from build123d import *

# Parameters (mm, degrees)
CROQUIS1_W              = 42.3
CROQUIS1_H              = 42.3
SALIENTE_EXTRUIR1_DEPTH = 7.6
SKETCH1_R               = 29.910616844
SKETCH1_R_2             = 27
CUT_EXTRUDE1_DEPTH      = 8.6
CROQUIS3_R              = 11
CROQUIS3_R_2            = 8.5
SALIENTE_EXTRUIR2_DEPTH = 2
CROQUIS4_R              = 4.5
CORTAR_EXTRUIR2_DEPTH   = 7
CROQUIS5_R              = 2.5
CORTAR_EXTRUIR3_DEPTH   = 7
CROQUIS6_R              = 1.5
CORTAR_EXTRUIR4_DEPTH   = 4.5
SKETCH2_R               = 5.5
CUT_EXTRUDE2_DEPTH      = 7.1
SKETCH3_R               = 16.5
SKETCH3_R_2             = 11.5
CUT_EXTRUDE3_DEPTH      = 0.1
FILLET1_R               = 1
FILLET2_R               = 0.5
CHAMFER1_SIZE           = 0.5


with BuildPart() as part:
    # Croquis1 → Saliente-Extruir1 (new body)
    with BuildSketch(Plane.XY):
        Rectangle(CROQUIS1_W, CROQUIS1_H)
    extrude(amount=SALIENTE_EXTRUIR1_DEPTH)

    # Sketch1 → Cut-Extrude1 (cut, through all)
    with BuildSketch(Plane(origin=(0, 0, 0), x_dir=(-1, 0, 0), z_dir=(0, 0, -1))):
        Circle(SKETCH1_R)
        Circle(SKETCH1_R_2, mode=Mode.SUBTRACT)
    extrude(amount=-CUT_EXTRUDE1_DEPTH, mode=Mode.SUBTRACT)

    # Croquis3 → Saliente-Extruir2 (add)
    with BuildSketch(Plane(origin=(0, 0, 0), x_dir=(-1, 0, 0), z_dir=(0, 0, -1))):
        Circle(CROQUIS3_R)
        Circle(CROQUIS3_R_2, mode=Mode.SUBTRACT)
    extrude(amount=SALIENTE_EXTRUIR2_DEPTH)

    # Croquis4 → Cortar-Extruir2 (cut)
    with BuildSketch(Plane(origin=(0, 0, -2), x_dir=(-1, 0, 0), z_dir=(0, 0, -1))):
        Circle(CROQUIS4_R)
    extrude(amount=-CORTAR_EXTRUIR2_DEPTH, mode=Mode.SUBTRACT)

    # Croquis5 → Cortar-Extruir3 (cut)
    with BuildSketch(Plane(origin=(0, 0, 5), x_dir=(-1, 0, 0), z_dir=(0, 0, -1))):
        Circle(CROQUIS5_R)
    extrude(amount=-CORTAR_EXTRUIR3_DEPTH, mode=Mode.SUBTRACT)

    # Croquis6 → Cortar-Extruir4 (cut)
    with BuildSketch(Plane(origin=(0, 0, 0), x_dir=(-1, 0, 0), z_dir=(0, 0, -1))):
        with Locations((-15.5, 15.5)):
            Circle(CROQUIS6_R)
        with Locations((15.5, 15.5)):
            Circle(CROQUIS6_R)
        with Locations((15.5, -15.5)):
            Circle(CROQUIS6_R)
        with Locations((-15.5, -15.5)):
            Circle(CROQUIS6_R)
    extrude(amount=-CORTAR_EXTRUIR4_DEPTH, mode=Mode.SUBTRACT)

    # Sketch2 → Cut-Extrude2 (cut)
    with BuildSketch(Plane.XY.offset(7.6)):
        Circle(SKETCH2_R)
    extrude(amount=-CUT_EXTRUDE2_DEPTH, mode=Mode.SUBTRACT)

    # Sketch3 → Cut-Extrude3 (cut)
    with BuildSketch(Plane(origin=(0, 0, 0), x_dir=(-1, 0, 0), z_dir=(0, 0, -1))):
        Circle(SKETCH3_R)
        Circle(SKETCH3_R_2, mode=Mode.SUBTRACT)
    extrude(amount=-CUT_EXTRUDE3_DEPTH, mode=Mode.SUBTRACT)

    # Fillet1
    fillet1_edges = [part.edges().sort_by_distance(p)[0] for p in [
        (21.15, 16.783250579, 3.8),
        (21.15, -16.783250579, 3.8),
        (-16.783250579, 21.15, 3.8),
        (16.783250579, 21.15, 3.8),
        (-21.15, -16.783250579, 3.8),
        (-21.15, 16.783250579, 3.8),
        (16.783250579, -21.15, 3.8),
        (-16.783250579, -21.15, 3.8),
    ]]
    fillet(fillet1_edges, radius=FILLET1_R)

    # Fillet2
    fillet2_edges = [part.edges().sort_by_distance(p)[0] for p in [
        (19.091883092, 19.091883092, 0),
        (0, 21.15, 0),
        (-21.15, 0, 0),
        (-19.091883092, 19.091883092, 0),
        (21.15, 0, 0),
        (19.091883092, -19.091883092, 0),
        (0, -21.15, 0),
        (-19.091883092, -19.091883092, 0),
        (-16.766402254, 21.092072184, 0),
        (-21.092072184, 16.766402254, 0),
        (-21.092072184, -16.766402254, 0),
        (-16.766402254, -21.092072184, 0),
        (16.766402254, -21.092072184, 0),
        (21.092072184, -16.766402254, 0),
        (21.092072184, 16.766402254, 0),
        (16.766402254, 21.092072184, 0),
    ]]
    fillet(fillet2_edges, radius=FILLET2_R)

    # Chamfer1
    chamfer1_edges = [part.edges().sort_by_distance(p)[0] for p in [
        (11, 0, -2),
    ]]
    chamfer(chamfer1_edges, length=CHAMFER1_SIZE)


solid = part.part
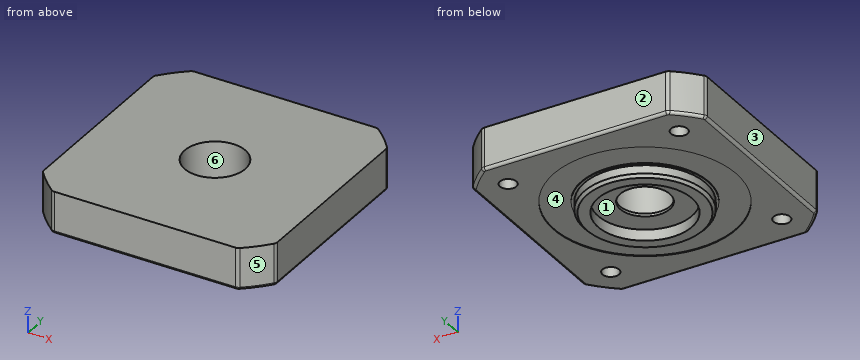
Could you check a few things on this model? Use its own coordinates, in mm. Face numbers are marked on the shaded views. A direction names the side the tool comes from. Give positions to 0.01 mm unless a question says otherwise; leave off trailing zeros. Order: outer loops, then holes, each group sorted by start corner. A loop starts at its lowest first (then second) coordinate and runs counter-clockwise, first axis right, second up. Notation, with made-up numbers: (11.25, -14.5) - (17.25, -14.5) arc R25 cw to (17.25, 17.5) - close; hole circle Ø5 at (58, 77.5). An arc over 180 degrees is marked (long way). One line per item, written item: value. Start each with the question number.
1. Imagine slicing it at C-C on y = -15. List the corners of the cut face in (x, z) for me, plus the area to 3 significant figures.
2. For P1, Ø8, axis at x = 0, y = 0, coming from the +Z side; P2, Ø2.5, axis at x = -16, y = -16, coming from the -Z side; P3, Ø2.5, axis at x = -15.5, y = -15.5, coming from the -Z side, each with a flat end and sliding along its axis, tell me the tip position at first contact or that it passes through.
3. For the marked faces 4, 5 and 6, which set-ups out of +Z, -Z, +X, -X, +Y, -Y let a thin tool reach every point of the face, with its end or its side?
4. Thinking about a two-plate mould opening in Y: for the marked faces 1, 2 and 3, which applies, +Y half, -Y half, draft (parallel to the pull), parting line (faces both ways), or undercut?
5. Imagine slicing it at D-D on z = -1. List the corners of the cut face in (x, y) for me.
6. Imagine slicing it at B-B on z = 4. List the corners of the cut face in (x, y) for me (3 decimals), plus the area to 3 significant figures.
7. If I drill on probe 1 along Y at (x, z) = (-15.5, 2.95); probe 2 along Y at (x, z) = (0, -1); probe 3 along Z at (x, y) = (-17, 13), over which ranges is the centre line in solid material (lowest first)?
Values:
1. outline: (-21.15, 0.5) arc R0.5 ccw to (-20.65, 0) - (-16.91, 0) - (-16.91, 4.5) - (-14.09, 4.5) - (-14.09, 0) - (-6.87, 0) - (-6.87, 0.1) - (6.87, 0.1) - (6.87, 0) - (14.09, 0) - (14.09, 4.5) - (16.91, 4.5) - (16.91, 0) - (20.65, 0) arc R0.5 ccw to (21.15, 0.5) - (21.15, 7.6) - (-21.15, 7.6) - close
1. area: 295 mm²
2. P1: through
2. P2: z = 0
2. P3: z = 4.5
3. face 4: -Z
3. face 5: +Z, -Z, +X, -Y
3. face 6: +Z
4. face 1: undercut
4. face 2: +Y half
4. face 3: draft
5. outline: circle Ø22 at (0, 0); hole circle Ø17 at (0, 0)
6. outline: (-21.15, -16.431) arc R1 ccw to (-20.925, -17.063) arc R27 ccw to (-17.063, -20.925) arc R1 ccw to (-16.431, -21.15) - (16.431, -21.15) arc R1 ccw to (17.063, -20.925) arc R27 ccw to (20.925, -17.063) arc R1 ccw to (21.15, -16.431) - (21.15, 16.431) arc R1 ccw to (20.925, 17.063) arc R27 ccw to (17.063, 20.925) arc R1 ccw to (16.431, 21.15) - (-16.431, 21.15) arc R1 ccw to (-17.063, 20.925) arc R27 ccw to (-20.925, 17.063) arc R1 ccw to (-21.15, 16.431) - close; hole circle Ø3 at (-15.5, -15.5); hole circle Ø3 at (-15.5, 15.5); hole circle Ø11 at (0, 0); hole circle Ø3 at (15.5, -15.5); hole circle Ø3 at (15.5, 15.5)
6. area: 1,630 mm²
7. probe 1: -21.15 to -17, -14 to 14, 17 to 21.15
7. probe 2: -11 to -8.5, 8.5 to 11
7. probe 3: 0 to 7.6
